Work out the finished part from the listing and answer in its coordinate system (mm). Round coordinates to 2 decimals unless told otherwise and drop trailing zeros. Loops run counter-clockwise (first coordinate to the right, second up) from the corner with the lowest first, then second, coordinate; pieces in that order, holes last. Notation, with made-up numbers: (10.5, -20) - (21.5, -20) arc R19 cw to (21.5, 2) - close; hole circle Ø5 at (65, 84). An arc over 180 degrees is marked (long way). Return JSON: item names as keys, results as strings.
from build123d import *

# Parameters (mm, degrees)
SKETCH1_R                           = 30.099
SKETCH1_R_2                         = 24.5618
BOSS_EXTRUDE1_DEPTH                 = 247.7
F_4_0MM_DOWEL_HOLE1_D               = 4
F_4_0MM_DOWEL_HOLE1_DEPTH           = 6
F_4_0MM_DOWEL_HOLE1_TIP             = 1.201721238
F_4_0MM_DOWEL_HOLE1_ON_FACE_2_D     = 4
F_4_0MM_DOWEL_HOLE1_ON_FACE_2_DEPTH = 6
F_4_0MM_DOWEL_HOLE1_ON_FACE_2_TIP   = 1.201721238
F_4_0MM_DOWEL_HOLE1_ON_FACE_3_D     = 4
F_4_0MM_DOWEL_HOLE1_ON_FACE_3_DEPTH = 6
F_4_0MM_DOWEL_HOLE1_ON_FACE_3_TIP   = 1.201721238
F_4_0MM_DOWEL_HOLE1_ON_FACE_4_D     = 4
F_4_0MM_DOWEL_HOLE1_ON_FACE_4_DEPTH = 6
F_4_0MM_DOWEL_HOLE1_ON_FACE_4_TIP   = 1.201721238
F_4_0MM_DOWEL_HOLE2_D               = 4
F_4_0MM_DOWEL_HOLE2_DEPTH           = 6
F_4_0MM_DOWEL_HOLE2_TIP             = 1.201721238
F_4_0MM_DOWEL_HOLE2_ON_FACE_2_D     = 4
F_4_0MM_DOWEL_HOLE2_ON_FACE_2_DEPTH = 6
F_4_0MM_DOWEL_HOLE2_ON_FACE_2_TIP   = 1.201721238
F_4_0MM_DOWEL_HOLE2_ON_FACE_3_D     = 4
F_4_0MM_DOWEL_HOLE2_ON_FACE_3_DEPTH = 6
F_4_0MM_DOWEL_HOLE2_ON_FACE_3_TIP   = 1.201721238
F_4_0MM_DOWEL_HOLE2_ON_FACE_4_D     = 4
F_4_0MM_DOWEL_HOLE2_ON_FACE_4_DEPTH = 6
F_4_0MM_DOWEL_HOLE2_ON_FACE_4_TIP   = 1.201721238


with BuildPart() as part:
    # Sketch1 → Boss-Extrude1 (new body)
    with BuildSketch(Plane.XY):
        Circle(SKETCH1_R)
        Circle(SKETCH1_R_2, mode=Mode.SUBTRACT)
    extrude(amount=BOSS_EXTRUDE1_DEPTH)

    # Ø4.0mm Dowel Hole1
    with Locations(Plane(origin=(0, 30.099, 7.5), x_dir=(1, 0, 0), z_dir=(0, 1, 0))):
        with Locations((0, 0)):
            Hole(F_4_0MM_DOWEL_HOLE1_D / 2, depth=F_4_0MM_DOWEL_HOLE1_DEPTH)
            with Locations((0, 0, -(F_4_0MM_DOWEL_HOLE1_DEPTH + F_4_0MM_DOWEL_HOLE1_TIP / 2))):  # 118° drill point
                Cone(0, F_4_0MM_DOWEL_HOLE1_D / 2, F_4_0MM_DOWEL_HOLE1_TIP, mode=Mode.SUBTRACT)

    # Ø4.0mm Dowel Hole1 on face 2
    with Locations(Plane(origin=(30.099, 0, 7.5), x_dir=(0, 0, 1), z_dir=(1, 0, 0))):
        with Locations((0, 0)):
            Hole(F_4_0MM_DOWEL_HOLE1_ON_FACE_2_D / 2, depth=F_4_0MM_DOWEL_HOLE1_ON_FACE_2_DEPTH)
            with Locations((0, 0, -(F_4_0MM_DOWEL_HOLE1_ON_FACE_2_DEPTH + F_4_0MM_DOWEL_HOLE1_ON_FACE_2_TIP / 2))):  # 118° drill point
                Cone(0, F_4_0MM_DOWEL_HOLE1_ON_FACE_2_D / 2, F_4_0MM_DOWEL_HOLE1_ON_FACE_2_TIP, mode=Mode.SUBTRACT)

    # Ø4.0mm Dowel Hole1 on face 3
    with Locations(Plane(origin=(0, -30.099, 7.5), x_dir=(0, 0, -1), z_dir=(0, -1, 0))):
        with Locations((0, 0)):
            Hole(F_4_0MM_DOWEL_HOLE1_ON_FACE_3_D / 2, depth=F_4_0MM_DOWEL_HOLE1_ON_FACE_3_DEPTH)
            with Locations((0, 0, -(F_4_0MM_DOWEL_HOLE1_ON_FACE_3_DEPTH + F_4_0MM_DOWEL_HOLE1_ON_FACE_3_TIP / 2))):  # 118° drill point
                Cone(0, F_4_0MM_DOWEL_HOLE1_ON_FACE_3_D / 2, F_4_0MM_DOWEL_HOLE1_ON_FACE_3_TIP, mode=Mode.SUBTRACT)

    # Ø4.0mm Dowel Hole1 on face 4
    with Locations(Plane(origin=(-30.099, 0, 7.5), x_dir=(0, 0, -1), z_dir=(-1, 0, 0))):
        with Locations((0, 0)):
            Hole(F_4_0MM_DOWEL_HOLE1_ON_FACE_4_D / 2, depth=F_4_0MM_DOWEL_HOLE1_ON_FACE_4_DEPTH)
            with Locations((0, 0, -(F_4_0MM_DOWEL_HOLE1_ON_FACE_4_DEPTH + F_4_0MM_DOWEL_HOLE1_ON_FACE_4_TIP / 2))):  # 118° drill point
                Cone(0, F_4_0MM_DOWEL_HOLE1_ON_FACE_4_D / 2, F_4_0MM_DOWEL_HOLE1_ON_FACE_4_TIP, mode=Mode.SUBTRACT)

    # Ø4.0mm Dowel Hole2
    with Locations(Plane(origin=(0, -30.099, 240.7), x_dir=(-1, 0, 0), z_dir=(0, -1, 0))):
        with Locations((0, 0)):
            Hole(F_4_0MM_DOWEL_HOLE2_D / 2, depth=F_4_0MM_DOWEL_HOLE2_DEPTH)
            with Locations((0, 0, -(F_4_0MM_DOWEL_HOLE2_DEPTH + F_4_0MM_DOWEL_HOLE2_TIP / 2))):  # 118° drill point
                Cone(0, F_4_0MM_DOWEL_HOLE2_D / 2, F_4_0MM_DOWEL_HOLE2_TIP, mode=Mode.SUBTRACT)

    # Ø4.0mm Dowel Hole2 on face 2
    with Locations(Plane(origin=(-30.099, 0, 240.7), x_dir=(0, 0, -1), z_dir=(-1, 0, 0))):
        with Locations((0, 0)):
            Hole(F_4_0MM_DOWEL_HOLE2_ON_FACE_2_D / 2, depth=F_4_0MM_DOWEL_HOLE2_ON_FACE_2_DEPTH)
            with Locations((0, 0, -(F_4_0MM_DOWEL_HOLE2_ON_FACE_2_DEPTH + F_4_0MM_DOWEL_HOLE2_ON_FACE_2_TIP / 2))):  # 118° drill point
                Cone(0, F_4_0MM_DOWEL_HOLE2_ON_FACE_2_D / 2, F_4_0MM_DOWEL_HOLE2_ON_FACE_2_TIP, mode=Mode.SUBTRACT)

    # Ø4.0mm Dowel Hole2 on face 3
    with Locations(Plane(origin=(0, 30.099, 240.7), x_dir=(0, 0, 1), z_dir=(0, 1, 0))):
        with Locations((0, 0)):
            Hole(F_4_0MM_DOWEL_HOLE2_ON_FACE_3_D / 2, depth=F_4_0MM_DOWEL_HOLE2_ON_FACE_3_DEPTH)
            with Locations((0, 0, -(F_4_0MM_DOWEL_HOLE2_ON_FACE_3_DEPTH + F_4_0MM_DOWEL_HOLE2_ON_FACE_3_TIP / 2))):  # 118° drill point
                Cone(0, F_4_0MM_DOWEL_HOLE2_ON_FACE_3_D / 2, F_4_0MM_DOWEL_HOLE2_ON_FACE_3_TIP, mode=Mode.SUBTRACT)

    # Ø4.0mm Dowel Hole2 on face 4
    with Locations(Plane(origin=(30.099, 0, 240.7), x_dir=(0, 0, 1), z_dir=(1, 0, 0))):
        with Locations((0, 0)):
            Hole(F_4_0MM_DOWEL_HOLE2_ON_FACE_4_D / 2, depth=F_4_0MM_DOWEL_HOLE2_ON_FACE_4_DEPTH)
            with Locations((0, 0, -(F_4_0MM_DOWEL_HOLE2_ON_FACE_4_DEPTH + F_4_0MM_DOWEL_HOLE2_ON_FACE_4_TIP / 2))):  # 118° drill point
                Cone(0, F_4_0MM_DOWEL_HOLE2_ON_FACE_4_D / 2, F_4_0MM_DOWEL_HOLE2_ON_FACE_4_TIP, mode=Mode.SUBTRACT)


solid = part.part
1) Flat-ended cylindrical pins translate along their axes: pin 1 (10 mm diameter, centred on x = -20.5, z = 104.5, fed in from +Y); pin 2 (10 mm diameter, centred on y = 10, z = 218.5, fed in from -X); pin 3 (5 mm diameter, centred on x = 3, z = 101.5, fed in from -Y); pin 4 (6.5 mm diameter, centred on y = 0, z = 240.7, fed in from -X). Find the tip coordinate at first contact, or state that the pin passes through.
Verdict:
{"pin 1": "stops at y = 25.8", "pin 2": "stops at x = -29.68", "pin 3": "stops at y = -30.09", "pin 4": "stops at x = -30.1"}
2) Section C-C (z = 67.5) is taken. Give the vertices of the cut face in (x, y).
Verdict:
{"outline": "circle Ø60.2 at (0, 0); hole circle Ø49.12 at (0, 0)"}
3) Find the intervals of material crossed by L1, parallel to Z at x = 0, y = -28.8; L2, parallel to Y at x = -1, z = 100; L3, parallel to Y at x = 0, z = 175, in increasing order.
Verdict:
{"L1": "z = 0 to 5.5, 9.5 to 238.7, 242.7 to 247.7", "L2": "y = -30.08 to -24.54, 24.54 to 30.08", "L3": "y = -30.1 to -24.56, 24.56 to 30.1"}
4) Section A-A (y = 5) is taken. Give the vertices of the cut face in (x, z).
Verdict:
{"outline": "(-29.68, 0) - (-24.05, 0) - (-24.05, 247.7) - (-29.68, 247.7) - close; (24.05, 0) - (29.68, 0) - (29.68, 247.7) - (24.05, 247.7) - close"}
5) Section B-B (x = -13) is taken. Give the vertices of the cut face in (y, z), and give its area (3 significant figures).
Verdict:
{"outline": "(-27.15, 0) - (-20.84, 0) - (-20.84, 247.7) - (-27.15, 247.7) - close; (20.84, 0) - (27.15, 0) - (27.15, 247.7) - (20.84, 247.7) - close", "area": "3,120 mm2"}
6) Determine the mould class of faces 1 (the flat face through (-25, 0, 0)), 2 (the cylindrical face through (-18.103, 16.6, 122.116)), 3 (the cylindrical face through (-0.434, -27.25, 242.652)), 4 (the cylindrical face through (-6.525, -29.383, 122.116)) for opening direction X: pulls with the +X half, pulls with the -X half, needs draft (parallel to the pull), parting line crosses it, or undercut.
Verdict:
{"face 1": "needs draft", "face 2": "undercut", "face 3": "undercut", "face 4": "parting line crosses it"}
